```python
from build123d import *

# Parameters (mm, degrees)
CHAMFER2_SIZE = 0.08


with BuildPart() as part:
    # Sketch1 → Revolve1 (revolve)
    with BuildSketch(Plane.XY):
        with BuildLine():
            Line((0.512347538, -3.1), (1.5, -3.1))
            Line((1.5, -3.1), (1.5, -2.5))
            Line((1.5, -2.5), (-1.5, -2.5))
            Line((-1.5, -2.5), (-1.5, -3.1))
            Line((-1.5, -3.1), (-0.512347538, -3.1))
            ThreePointArc((-0.512347538, -3.1), (0, -2.85), (0.512347538, -3.1))
        make_face()
    revolve(axis=Axis((-6.429017492, 0, 0), (1, 0, 0)))

    # Chamfer2
    chamfer2_edges = [part.edges().sort_by_distance(p)[0] for p in [
        (1.5, 3.1, 0),
        (1.5, 2.5, 0),
        (-1.5, 2.5, 0),
        (-1.5, 3.1, 0),
    ]]
    chamfer(chamfer2_edges, length=CHAMFER2_SIZE)


solid = part.part
```
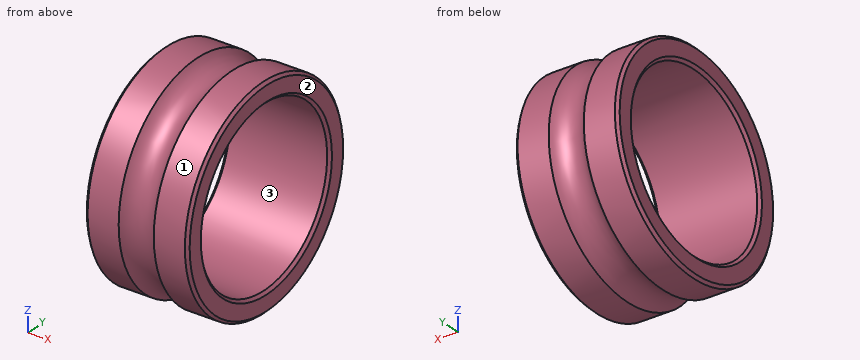
Source: CAD feature listing. Evaluate the final solid. Frame: model axes, mm. Face numbers are marked on the shaded views. Round coordinates to 2 decimals unless told otherwise and drop trailing zeros. Loops run counter-clockwise (first coordinate to the right, second up) from the corner with the lowest first, then second, coordinate; pieces in that order, holes last. Notation, with made-up numbers: M 76,12.5 L 108,12.5 A14 ccw 108,33.5 Z; hole C 12,-23 d3. An arc over 180 degrees is marked long. Use a Markdown table: item, result. Add a question column.
1. Ray query, line 1 along Z through (x, y) = (0.7, 0); line 2 along Y through (x, z) = (1.3, -0.5). Return the intervals inside material, ascending. Write a range as [from, to].
2. Cut plane A-A, the plane y = 0. Output: boundary loops of the cut face in (x, z).
3. Cut plane C-C, the plane x = -1.2. Output: boundary loops of the cut face in (y, z), and give its area (3 significant figures).
4. Contact query for flat-ended pins moving along their axis: pin 1 (1.5 mm diameter, centred on x = -0.5, y = 2.5, fed in from -Z); pin 2 (1.5 mm diameter, centred on x = -1, y = -1, fed in from -Z). Output: stop coordinate, or through.
5. Pull-direction query (Z, two-part tool) for the marked faces 1, 2 and 3; classes: +Z half, -Z half, draft (parallel to the pull), parting line (faces both ways), or undercut.
6. Cut plane D-D, the plane x = 0.2. Output: boundary loops of the cut face in (y, z).
Solution:
| question | item | result |
|---|---|---|
| 1 | line 1 | z = [-3.1, -2.5], [2.5, 3.1] |
| 1 | line 2 | y = [-3.06, -2.45], [2.45, 3.06] |
| 2 | outline | M -1.5,-3.02 L -1.42,-3.1 L -0.51,-3.1 A0.65 cw 0.51,-3.1 L 1.42,-3.1 L 1.5,-3.02 L 1.5,-2.58 L 1.42,-2.5 L -1.42,-2.5 L -1.5,-2.58 Z; M -1.5,2.58 L -1.42,2.5 L 1.42,2.5 L 1.5,2.58 L 1.5,3.02 L 1.42,3.1 L 0.51,3.1 A0.65 cw -0.51,3.1 L -1.42,3.1 L -1.5,3.02 Z |
| 3 | outline | C 0,0 d6.2; hole C 0,0 d5 |
| 3 | area | 10.6 mm2 |
| 4 | pin 1 | stops at z = -2.56 |
| 4 | pin 2 | stops at z = -3.09 |
| 5 | face 1 | parting line |
| 5 | face 2 | draft |
| 5 | face 3 | undercut |
| 6 | outline | C 0,0 d5.76; hole C 0,0 d5 |
